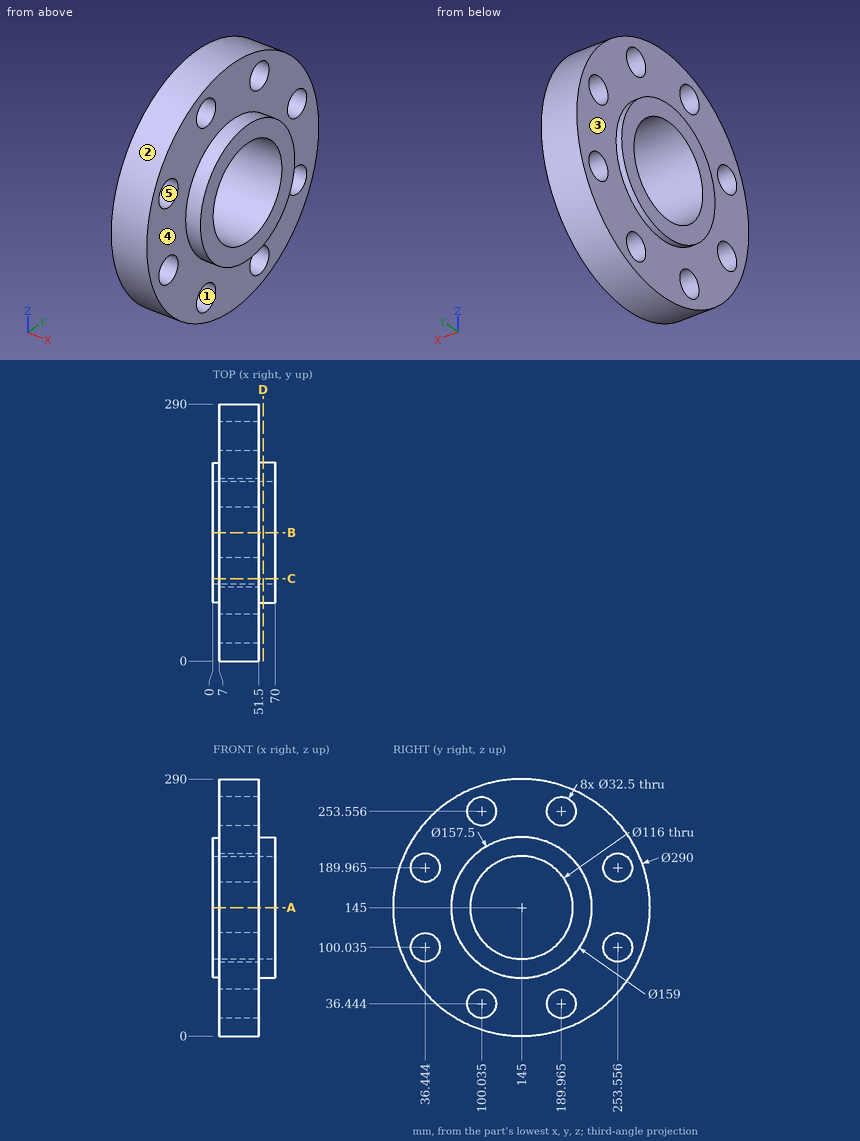
Could you check a few things on this drawing? It's one solid part, dimensions in mm from its lowest x, y, z. A direction names the side the tool comes from. Round coordinates to 2 decimals unless told otherwise and drop trailing zeros. Loops run counter-clockwise (first coordinate to the right, second up) from the corner with the lowest first, then second, coordinate; pieces in that order, holes last.
Q1. I want a section at C-C (y = 93). Write out the boundary of the cut face in (x, z) (1 decimal).
Q2. For P1, Ø5, axis at x = 50.5, z = 73, coming from the +Y side; P2, Ø1.5, axis at x = 35.5, y = 157.5, coming from the -Z side; P3, Ø1.5, axis at x = 28.5, z = 63.5, coming from the -Y side (1 decimal), each with a flat end and sliding along its axis, tell me the tip position at first contact or that it passes through.
Q3. On a 3-axis mill with a long thin cutter (end or side, diameter ignored), from which of +Z, -Z, +X, -X, +Y, -Y can I reach the whole of each face in a straight line? I mean the marked faces 4 and 5. Say none if no direction works.
Q4. I want a section at D-D (x = 56.5). Write out the boundary of the cut face in (y, z).
Q5. Please list where these lines run through material, in increasing order: L1, parallel to Y at x = 44.5, z = 184; L2, parallel to Y at x = 48.5, z = 100 (1 decimal); L3, parallel to Y at x = 23.5, z = 25 (1 decimal).
Q6. Thinking about a two-plate mould opening in Y: for the marked faces 1, 2 and 3, which applies, pulls with the +Y half, pulls with the -Y half, needs draft (parallel to the pull), parting line crosses it, or undercut?
Q7. I want a section at A-A (z = 145). Write out the boundary of the cut face in (x, y), and give its area (3 significant figures).
Answer below:
1. outline: (0, 85.9) - (7, 85.9) - (7, 51.1) - (51.5, 51.1) - (51.5, 84.9) - (70, 84.9) - (70, 119.3) - (0, 119.3) - close; (0, 170.7) - (70, 170.7) - (70, 205.1) - (51.5, 205.1) - (51.5, 238.9) - (7, 238.9) - (7, 204.1) - (0, 204.1) - close; (7, 9.6) - (51.5, 9.6) - (51.5, 21.8) - (7, 21.8) - close; (7, 268.2) - (51.5, 268.2) - (51.5, 280.4) - (7, 280.4) - close
2. P1: stops at y = 272.26
2. P2: stops at z = 0.48
2. P3: stops at y = 24.6
3. face 4: +X
3. face 5: +X, -X
4. outline: circle Ø159 at (145, 145); hole circle Ø116 at (145, 145)
5. L1: y = 5.34 to 21.33, 51.56 to 102.07, 187.93 to 238.44, 268.67 to 284.66
5. L2: y = 7.2 to 20.2, 52.7 to 108.4, 181.6 to 237.3, 269.8 to 282.8
5. L3: y = 63.6 to 88.5, 111.6 to 178.4, 201.5 to 226.4
6. face 1: undercut
6. face 2: parting line crosses it
6. face 3: needs draft
7. outline: (0, 66.25) - (7, 66.25) - (7, 0) - (51.5, 0) - (51.5, 65.5) - (70, 65.5) - (70, 87) - (0, 87) - close; (0, 203) - (70, 203) - (70, 224.5) - (51.5, 224.5) - (51.5, 290) - (7, 290) - (7, 223.75) - (0, 223.75) - close
7. area: 8,830 mm2
